from build123d import *

# Parameters (mm, degrees)
BOSS_EXTRUDE1_DEPTH          = 450
SKETCH3_R                    = 30
CUT_EXTRUDE2_DEPTH           = 609.050936432
M10_CLEARANCE_SLOT1_D        = 11
CUT_EXTRUDE_THIN4_DEPTH      = 609.050936432
CUT_EXTRUDE_THIN4_DEPTH_BACK = 0.1
CUT_EXTRUDE_THIN5_DEPTH      = 609.050936432
CUT_EXTRUDE_THIN5_DEPTH_BACK = 0.1
CUT_EXTRUDE_THIN6_DEPTH      = 609.050936432
CUT_EXTRUDE_THIN6_DEPTH_BACK = 0.1


with BuildPart() as part:
    # Sketch1 → Boss-Extrude1 (new body)
    with BuildSketch(Plane.XY):
        with BuildLine():
            Line((-96.40006218, 31.988224321), (-96.40006218, -14.011775679))
            ThreePointArc((-96.40006218, -14.011775679), (-95.521382524, -16.133096022), (-93.40006218, -17.011775679))
            Line((-93.40006218, -17.011775679), (96.59993782, -17.011775679))
            ThreePointArc((96.59993782, -17.011775679), (98.721258163, -16.133096022), (99.59993782, -14.011775679))
            Line((99.59993782, -14.011775679), (99.59993782, 31.988224321))
            Line((99.59993782, 31.988224321), (102.59993782, 31.988224321))
            Line((102.59993782, 31.988224321), (102.59993782, -17.011775679))
            ThreePointArc((102.59993782, -17.011775679), (101.721258163, -19.133096022), (99.59993782, -20.011775679))
            Line((99.59993782, -20.011775679), (-96.40006218, -20.011775679))
            ThreePointArc((-96.40006218, -20.011775679), (-98.521382524, -19.133096022), (-99.40006218, -17.011775679))
            Line((-99.40006218, -17.011775679), (-99.40006218, 31.988224321))
            Line((-99.40006218, 31.988224321), (-96.40006218, 31.988224321))
        make_face()
    extrude(amount=BOSS_EXTRUDE1_DEPTH)

    # Sketch3 → Cut-Extrude2 (cut, through all)
    with BuildSketch(Plane(origin=(-323.698265728, -20.011775679, 19.544679499), x_dir=(0, 0, -1), z_dir=(0, -1, 0))):
        with Locations((-325.455320501, 287.298203547)):
            Circle(SKETCH3_R)
    extrude(amount=-CUT_EXTRUDE2_DEPTH, mode=Mode.SUBTRACT)

    # M10 Clearance Slot1 (through all)
    with Locations(Plane(origin=(-323.698265728, -20.011775679, 19.544679499), x_dir=(0, 0, -1), z_dir=(0, -1, 0))):
        with Locations((-380.455320501, 390.298203547), (-205.455320501, 390.298203547), (-30.455320501, 390.298203547), (-30.455320501, 259.298203547), (-205.455320501, 259.298203547), (-380.455320501, 259.298203547)):
            Hole(M10_CLEARANCE_SLOT1_D / 2)

    # Sketch9 → Cut-Extrude-Thin4 (cut, two sides: drawn at the far end of the back side and taken through both)
    with BuildSketch(Plane(origin=(-323.698265728, -20.011775679, 19.544679499), x_dir=(0, 0, -1), z_dir=(0, -1, 0)).offset(-CUT_EXTRUDE_THIN4_DEPTH_BACK)):
        Polygon((-307.687440193, 227.298203547), (-307.687440193, 262.63145603), (-256.25354627, 262.63145603), (-256.25354627, 227.298203547), (-256.15354627, 227.298203547), (-256.15354627, 262.73145603), (-307.787440193, 262.73145603), (-307.787440193, 227.298203547), align=None)
    extrude(amount=CUT_EXTRUDE_THIN4_DEPTH + CUT_EXTRUDE_THIN4_DEPTH_BACK, mode=Mode.SUBTRACT)

    # Sketch10 → Cut-Extrude-Thin5 (cut, two sides: drawn at the far end of the back side and taken through both)
    with BuildSketch(Plane(origin=(-323.698265728, -20.011775679, 19.544679499), x_dir=(0, 0, -1), z_dir=(0, -1, 0)).offset(-CUT_EXTRUDE_THIN5_DEPTH_BACK)):
        Polygon((-69.477840086, 227.298203547), (-69.477840086, 262.740474595), (-120.654750778, 262.740474595), (-120.654750778, 227.298203547), (-120.554750778, 227.298203547), (-120.554750778, 262.640474595), (-69.577840086, 262.640474595), (-69.577840086, 227.298203547), align=None)
    extrude(amount=CUT_EXTRUDE_THIN5_DEPTH + CUT_EXTRUDE_THIN5_DEPTH_BACK, mode=Mode.SUBTRACT)

    # Sketch11 → Cut-Extrude-Thin6 (cut, two sides: drawn at the far end of the back side and taken through both)
    with BuildSketch(Plane(origin=(-323.698265728, -20.011775679, 19.544679499), x_dir=(0, 0, -1), z_dir=(0, -1, 0)).offset(-CUT_EXTRUDE_THIN6_DEPTH_BACK)):
        Polygon((-162.791670666, 423.298203547), (-162.791670666, 403.614782025), (-214.233995463, 403.614782025), (-214.233995463, 423.298203547), (-214.333995463, 423.298203547), (-214.333995463, 403.514782025), (-162.691670666, 403.514782025), (-162.691670666, 423.298203547), align=None)
    extrude(amount=CUT_EXTRUDE_THIN6_DEPTH + CUT_EXTRUDE_THIN6_DEPTH_BACK, mode=Mode.SUBTRACT)


solid = part.part
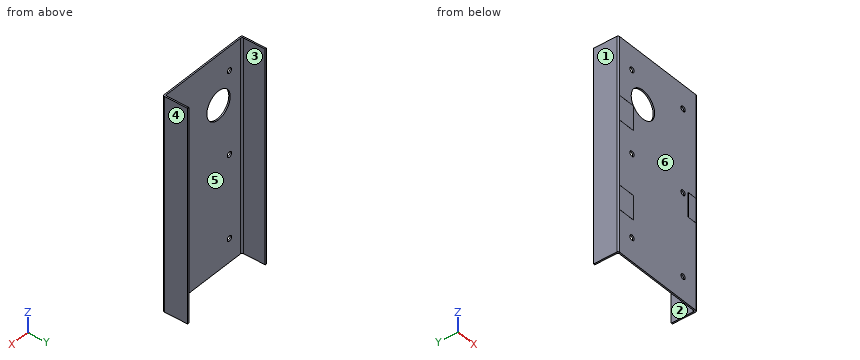
Model file for the job. Use its own axes, mm. Face numbers are marked on the shaded views. A direction names the side the tool comes from. Round coordinates to 2 decimals unless told otherwise and drop trailing zeros. Order: outer loops, then holes, each group sorted by start corner. A loop starts at its lowest first (then second) coordinate and runs counter-clockwise, first axis right, second up. Notation, with made-up numbers: M 55,52 L 98,52 A21 ccw 98,77 Z; hole C -30,22 d9. An arc over 180 degrees is marked long. Write each question's results on one line, items separated by ' | '. Start each with the question number.
(1) Saw through at B-B, the plane y = 15. Give the cut face in (x, z).
(2) Saw through at A-A, the plane z = 225. Give the cut face in (x, y), then the cut area to 3 significant figures.
(3) Drop a flat-ended pin along its axis: pin 1 (3 mm diameter, centred on x = 57, z = 54, fed in from +Y). Give the stop position or say it passes through.
(4) Probe probe 1 along X at (y, z) = (-17.7, 225); probe 2 along X at (y, z) = (15.5, 377.5); probe 3 along X at (y, z) = (-18.35, 400). List the from-to ranges inside material, lowest first. Write a range as from..to.
(5) Which spindle directions (+Z, -Z, +X, -X, +Y, -Y) get a long thin tool onto all of the face, cutting with end or side? Do the marked faces 1 and 2. Say none if no direction does.
(6) Two-plate mould, pull along X, no slides. Class the marked faces 3, 4, 5 and 6: pulls with the +X half, pulls with the -X half, needs draft (parallel to the pull), parting line crosses it, or undercut.
(7) Saw through at C-C, the plane z = 345. Give the cut face in (x, y), then the cut area to 3 significant figures.
(8) Saw through at D-D, the plane x = 85.5. Give the cut face in (y, z), then the cut area to 3 significant figures.
Established:
1) outline: M -99.4,0 L -96.4,0 L -96.4,450 L -99.4,450 Z; M 99.6,0 L 102.6,0 L 102.6,450 L 99.6,450 Z
2) outline: M -99.4,-17.01 A3 ccw -96.4,-20.01 L -69.9,-20.01 L -69.9,-17.01 L -93.4,-17.01 A3 cw -96.4,-14.01 L -96.4,31.99 L -99.4,31.99 Z; M -58.9,-20.01 L 61.1,-20.01 L 61.1,-17.01 L -58.9,-17.01 Z; M 72.1,-20.01 L 79.82,-20.01 L 79.82,-19.91 L 79.92,-19.91 L 79.92,-20.01 L 99.6,-20.01 A3 ccw 102.6,-17.01 L 102.6,31.99 L 99.6,31.99 L 99.6,-14.01 A3 cw 96.6,-17.01 L 72.1,-17.01 Z | area: 834 mm^2
3) pin 1: stops at y = -17.01
4) probe 1: x = -99.32..-69.9, -58.9..61.1, 72.1..102.52 | probe 2: x = -99.4..-96.4, 99.6..102.6 | probe 3: x = -99.09..-69.9, -58.9..61.1, 72.1..102.28
5) face 1: +Z, -Z, -X, +Y, -Y | face 2: +Z, -Z, +Y
6) face 3: undercut | face 4: pulls with the +X half | face 5: undercut | face 6: needs draft
7) outline: M -99.4,-17.01 A3 ccw -96.4,-20.01 L -66.4,-20.01 L -66.4,-17.01 L -93.4,-17.01 A3 cw -96.4,-14.01 L -96.4,31.99 L -99.4,31.99 Z; M -6.4,-20.01 L 99.6,-20.01 A3 ccw 102.6,-17.01 L 102.6,31.99 L 99.6,31.99 L 99.6,-14.01 A3 cw 96.6,-17.01 L -6.4,-17.01 Z | area: 720 mm^2
8) outline: M -20.01,0 L -17.01,0 L -17.01,450 L -20.01,450 L -20.01,233.88 L -19.91,233.88 L -19.91,233.78 L -20.01,233.78 L -20.01,182.34 L -19.91,182.34 L -19.91,182.24 L -20.01,182.24 Z | area: 1,350 mm^2
